```python
from build123d import *

# Parameters (mm, degrees)
SCHNITT_LINEAR_AUSTRAGEN1_DEPTH = 1
FASE1_SIZE                      = 0.2


with BuildPart() as part:
    # Skizze1 → Rotation1 (revolve)
    with BuildSketch(Plane(origin=(0, 0, 0), x_dir=(0, 0, -1), z_dir=(1, 0, 0))):
        Polygon((0, 0), (0, 2.9), (0.6, 2.9), (2, 1.5), (5, 1.5), (5, 0), align=None)
    revolve(axis=Axis((0, 0, 31.763581507), (0, 0, -1)))

    # Skizze3 → Schnitt-Linear austragen1 (cut)
    with BuildSketch(Plane.XY):
        Polygon((1, -0.577350269), (1, 0.577350269), (0, 1.154700538), (-1, 0.577350269), (-1, -0.577350269), (0, -1.154700538), align=None)
    extrude(amount=-SCHNITT_LINEAR_AUSTRAGEN1_DEPTH, mode=Mode.SUBTRACT)

    # Fase1
    fase1_edges = [part.edges().sort_by_distance(p)[0] for p in [
        (0, -1.5, -5),
    ]]
    chamfer(fase1_edges, length=FASE1_SIZE)


solid = part.part
```
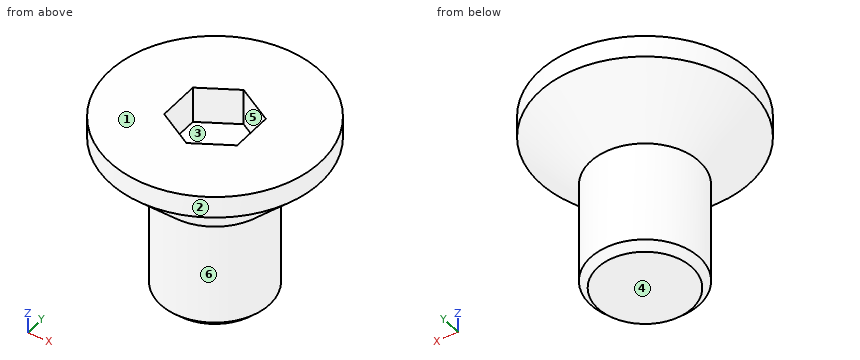
Geometry: final body of the model. Coordinates: model frame, mm. Face numbers are marked on the shaded views. A direction names the side the tool comes from. Round coordinates to 2 decimals unless told otherwise and drop trailing zeros. Loops run counter-clockwise (first coordinate to the right, second up) from the corner with the lowest first, then second, coordinate; pieces in that order, holes last.
Item 1: Section C-C, the plane z = -3.15. Output: boundary loops of the cut face in (x, y).
Checked values:
outline: circle Ø3 at (0, 0)
Item 2: Contact query for flat-ended pins moving along their axis: P1, Ø3, axis at x = -1.5, y = 1.5, coming from the -Z side; P2, Ø0.6, axis at x = 0, y = 0, coming from the +Z side; P3, Ø1, axis at y = 1, z = -4.5, coming from the -X side. Output: stop coordinate, or through.
Checked values:
P1: stops at z = -5
P2: stops at z = -1
P3: stops at x = -1.41
Item 3: Section A-A, the plane y = 0. Output: boundary loops of the cut face in (x, z).
Checked values:
outline: (-2.9, -0.6) - (-1.5, -2) - (-1.5, -4.8) - (-1.3, -5) - (1.3, -5) - (1.5, -4.8) - (1.5, -2) - (2.9, -0.6) - (2.9, 0) - (1, 0) - (1, -1) - (-1, -1) - (-1, 0) - (-2.9, 0) - close
Item 4: Reachability of the marked faces 4, 5 and 6 from +Z, -Z, +X, -X, +Y, -Y: full face, straight path, thin tool, end or side. Return the list, or none.
Checked values:
face 4: -Z, +X, -X, +Y, -Y
face 5: +Z
face 6: -Z
Item 5: Line query: L1, parallel to X at y = -1.1, z = -0.15; L2, parallel to X at y = 1, z = -3.7; L3, parallel to Y at x = -0.4, z = -2.2. Output: solid intervals per line, ascending.
Checked values:
L1: x = -2.68 to -0.09, 0.09 to 2.68
L2: x = -1.12 to 1.12
L3: y = -1.45 to 1.45
Item 6: Section B-B, the plane z = -1.2. Output: boundary loops of the cut face in (x, y), plus the area to 3 significant figures.
Checked values:
outline: circle Ø4.6 at (0, 0)
area: 16.6 mm2
Item 7: Mould query, pull axis X, two halves, no side actions, for the marked faces 1, 2 and 3. Classes: released by +X, released by -X, zero draft, split by the parting line, or undercut.
Checked values:
face 1: zero draft
face 2: split by the parting line
face 3: undercut
